Read the model definition and answer for the solid it produces. Units are mm, in the model's axes. A direction names the side the tool comes from. Coordinates: 2 decimals unless noted, no trailing zeros. Loops run counter-clockwise (first coordinate to the right, second up) from the corner with the lowest first, then second, coordinate; pieces in that order, holes last.
from build123d import *

# Parameters (mm, degrees)
BOSS_EXTRUDE1_DEPTH = 6.35
SKETCH2_W           = 19.05
SKETCH2_H           = 6.35
CUT_EXTRUDE1_DEPTH  = 131.484388434


with BuildPart() as part:
    # Sketch1 → Boss-Extrude1 (new body)
    with BuildSketch(Plane.XY):
        Polygon((107.95, 3.175), (107.95, 9.525), (101.6, 9.525), (101.6, 60.325), (107.95, 60.325), (107.95, 66.675), (95.25, 66.675), (95.25, 73.025), (-44.45, 73.025), (-44.45, 66.675), (-57.15, 66.675), (-57.15, 60.325), (-50.8, 60.325), (-50.8, 9.525), (-57.15, 9.525), (-57.15, 3.175), (-44.45, 3.175), (-44.45, -3.175), (95.25, -3.175), (95.25, 3.175), align=None)
    extrude(amount=-BOSS_EXTRUDE1_DEPTH)

    # Sketch2 → Cut-Extrude1 (cut, through all)
    with BuildSketch(Plane.XY):
        with Locations((98.425, 57.15)):
            Rectangle(SKETCH2_W, SKETCH2_H)
        with Locations((-47.625, 57.15)):
            Rectangle(SKETCH2_W, SKETCH2_H)
    extrude(amount=-CUT_EXTRUDE1_DEPTH, mode=Mode.SUBTRACT)


solid = part.part
Q1. Determine the mould class of faces 5 (the face through (24, -3.175, -3)), 6 (the face through (-50.8, 32, -3)), 7 (the face through (95.25, 0, -3)), 8 (the face through (-45, 53.975, -3)) for opening direction Y: +Y half, -Y half, draft (parallel to the pull), parting line (faces both ways), or undercut.
Findings below:
face 5: -Y half
face 6: undercut
face 7: draft
face 8: undercut
Q2. Flat-ended cylindrical pins translate along their axes: pin 1 Ø1.9 at (y, z) = (71, -3.5) entering from -X; pin 2 Ø10 at (x, y) = (50.5, 9) entering from +Z; pin 3 Ø3 at (y, z) = (56.5, -1) entering from -X; pin 4 Ø2 at (y, z) = (38, -1.5) entering from +X. Find the tip coordinate at first contact, or state that the pin passes through.
Findings below:
pin 1: stops at x = -44.45
pin 2: stops at z = 0
pin 3: stops at x = -38.1
pin 4: stops at x = 101.6
Q3. Which of the six approach directions +Z, -Z, +X, -X, +Y, -Y give full straight-line access (tool end or side, diameter ignored) to faces 1 (the face through (102, 3.175, -3)), 2 (the face through (-51, 3.175, -3)), 3 (the face through (-38.1, 57, -3)), 4 (the face through (102, 66.675, -3))?
Findings below:
face 1: +Z, -Z, +X, -Y
face 2: +Z, -Z, -X, -Y
face 3: +Z, -Z, -X
face 4: +Z, -Z, +X, +Y
Q4. A cutting plane is placed at A-A (z = -1). Give the vertices of the cut face in (x, y) (3 decimals).
Findings below:
outline: (-57.15, 3.175) - (-44.45, 3.175) - (-44.45, -3.175) - (95.25, -3.175) - (95.25, 3.175) - (107.95, 3.175) - (107.95, 9.525) - (101.6, 9.525) - (101.6, 53.975) - (88.9, 53.975) - (88.9, 60.325) - (107.95, 60.325) - (107.95, 66.675) - (95.25, 66.675) - (95.25, 73.025) - (-44.45, 73.025) - (-44.45, 66.675) - (-57.15, 66.675) - (-57.15, 60.325) - (-38.1, 60.325) - (-38.1, 53.975) - (-50.8, 53.975) - (-50.8, 9.525) - (-57.15, 9.525) - close
Q5. A cutting plane is placed at B-B (y = 34). Give the vertices of the cut face in (x, z).
Findings below:
outline: (-50.8, -6.35) - (101.6, -6.35) - (101.6, 0) - (-50.8, 0) - close
Q6. Straight lines are drawn through the part: probe 1 along Y at (x, z) = (-43, -0.5) (3 decimals); probe 2 along X at (y, z) = (30, -5.25); probe 3 along X at (y, z) = (69, -2.25). For each, find the intervals that lie inside material, in ascending order.
Findings below:
probe 1: y = -3.175 to 53.975, 60.325 to 73.025
probe 2: x = -50.8 to 101.6
probe 3: x = -44.45 to 95.25
